from build123d import *

# Parameters (mm, degrees)
BOSS_EXTRUDE1_DEPTH = 12.7
SKETCH2_W           = 44.45
SKETCH2_H           = 19.05
CUT_EXTRUDE1_DEPTH  = 100.3932216


with BuildPart() as part:
    # Sketch1 → Boss-Extrude1 (new, symmetric)
    with BuildSketch(Plane.XY):
        Polygon((-25.4, -47.625), (25.4, -47.625), (25.4, 34.925), (12.7, 34.925), (12.7, 47.625), (-25.4, 3.175), align=None)
    extrude(amount=BOSS_EXTRUDE1_DEPTH, both=True)

    # Sketch2 → Cut-Extrude1 (cut, through all)
    with BuildSketch(Plane.XZ.offset(47.625)):
        Rectangle(SKETCH2_W, SKETCH2_H)
    extrude(amount=-CUT_EXTRUDE1_DEPTH, mode=Mode.SUBTRACT)


solid = part.part
Input: part model. Units: mm. Frame: model coordinates. A direction names the side the tool comes from. Give positions to 0.01 mm unless a question says otherwise; leave off trailing zeros. Order: outer loops, then holes, each group sorted by start corner. A loop starts at its lowest first (then second) coordinate and runs counter-clockwise, first axis right, second up. Notation, with made-up numbers: (-14, 71.5) - (3, 71.5) arc R27 cw to (3, 106.5) - close; hole circle Ø11 at (36, -35.75). An arc over 180 degrees is marked (long way). Write each question's results on one line, items separated by ' | '.
Item 1: Contact query for flat-ended pins moving along their axis: pin 1 Ø12 at (x, z) = (17, 5) entering from -Y (3 decimals); pin 2 Ø12 at (x, z) = (-15.5, -9) entering from +Y; pin 3 Ø1 at (y, z) = (41, -11.5) entering from +X. Output: stop coordinate, or through.
A:
pin 1: stops at y = -47.625 | pin 2: stops at y = 21.7 | pin 3: stops at x = 12.7
Item 2: Access query for faces 4 (the flat face through (12.7, 41, 11)), 5 (the flat face through (-10.494, 20.565, -10.289)), 6 (the flat face through (0, -11, 9.525)). Directions: +Z, -Z, +X, -X, +Y, -Y. A direction counts if a zero-diameter tool reaches every point of the face in a straight line with its end or side. Return the directions, or none.
A:
face 4: +Z, -Z, +X, +Y | face 5: +Z, -Z, -X, +Y | face 6: +Y, -Y
Item 3: Section A-A (z = 6.5). Return loops of the section in (x, y) (3 decimals).
A:
outline: (-25.4, -47.625) - (-22.225, -47.625) - (-22.225, 6.879) - (-25.4, 3.175) - close; (22.225, -47.625) - (25.4, -47.625) - (25.4, 34.925) - (22.225, 34.925) - close
Item 4: Section D-D (z = -10.75). Return loops of the section in (x, y) (3 decimals).
A:
outline: (-25.4, -47.625) - (25.4, -47.625) - (25.4, 34.925) - (12.7, 34.925) - (12.7, 47.625) - (-25.4, 3.175) - close
Item 5: Draft query along X for faces 1 (the flat face through (22.225, -7, 0)), 2 (the flat face through (0, -10, -12.7)), 3 (the flat face through (25.4, -7, 0)). Return one class per face: released by +X, released by -X, zero draft, split by the parting line, or undercut.
A:
face 1: undercut | face 2: zero draft | face 3: released by +X
Item 6: Section C-C (x = -5.5). Return loops of the section in (y, z) (3 decimals).
A:
outline: (-47.625, -12.7) - (26.392, -12.7) - (26.392, -9.525) - (-47.625, -9.525) - close; (-47.625, 9.525) - (26.392, 9.525) - (26.392, 12.7) - (-47.625, 12.7) - close
Item 7: Material intervals for line 1 along Z through (x, y) = (6, -12) (3 decimals); line 2 along X through (y, z) = (-3, 8) (3 decimals); line 3 along X through (y, z) = (18, -2.75) (3 decimals), sorted ascending.
A:
line 1: z = -12.7 to -9.525, 9.525 to 12.7 | line 2: x = -25.4 to -22.225, 22.225 to 25.4 | line 3: x = 22.225 to 25.4
Item 8: Section B-B (y = -40.5). Return loops of the section in (x, z) (3 decimals), and give its area (3 significant figures).
A:
outline: (-25.4, -12.7) - (25.4, -12.7) - (25.4, 12.7) - (-25.4, 12.7) - close; hole (-22.225, -9.525) - (22.225, -9.525) - (22.225, 9.525) - (-22.225, 9.525) - close | area: 444 mm^2
